from build123d import *

# Parameters (mm, degrees)
SKETCH1_W           = 1.905
SKETCH1_H           = 10.16
BOSS_EXTRUDE2_DEPTH = 3.175
SKETCH2_R           = 1.27
CUT_EXTRUDE1_DEPTH  = 52.07


with BuildPart() as part:
    # Sketch1 → Boss-Extrude2 (new body)
    with BuildSketch(Plane(origin=(0, 0, 0), x_dir=(1, 0, 0), z_dir=(0, 1, 0))):
        Polygon((-1.5875, 25.4), (-1.5875, -25.4), (1.5875, -25.4), (1.5875, 25.4), (1.5875, 38.1), (-1.5875, 38.1), align=None)
        with Locations((0, 31.75)):
            Rectangle(SKETCH1_W, SKETCH1_H, mode=Mode.SUBTRACT)
    extrude(amount=BOSS_EXTRUDE2_DEPTH)

    # Sketch2 → Cut-Extrude1 (cut)
    with BuildSketch(Plane.XY.offset(25.4)):
        with Locations((0, 1.5875)):
            Circle(SKETCH2_R)
    extrude(amount=-CUT_EXTRUDE1_DEPTH, mode=Mode.SUBTRACT)


solid = part.part
CAD build for the part. Positions are in the model's coordinates, mm. A direction names the side the tool comes from. Round coordinates to 2 decimals unless told otherwise and drop trailing zeros. Order: outer loops, then holes, each group sorted by start corner. A loop starts at its lowest first (then second) coordinate and runs counter-clockwise, first axis right, second up. Notation, with made-up numbers: (83, 17.5) - (104, 17.5) arc R15 cw to (104, 24.5) - close; hole circle Ø4 at (-18, 88). An arc over 180 degrees is marked (long way). Return JSON: item names as keys, results as strings.
(1) Cut at B-B (z = 18.5). Give the cut face in (x, y) (1 decimal).
Answer key:
{"outline": "(-1.6, 0) - (1.6, 0) - (1.6, 3.2) - (-1.6, 3.2) - close; hole circle Ø2.5 at (0, 1.6)"}
(2) Wall check: probe 1 along X at (y, z) = (0.75, -14); probe 2 along Y at (x, z) = (0, 6.5) (1 decimal); probe 3 along X at (y, z) = (1.65, -8.5). Give the ranges that are in metal, low to high. Write a range as from..to.
Answer key:
{"probe 1": "x = -1.59..-0.95, 0.95..1.59", "probe 2": "y = 0..0.3, 2.9..3.2", "probe 3": "x = -1.59..-1.27, 1.27..1.59"}
(3) Cut at A-A (x = 0). State how many separate pieces and enclosed holes the cut face has, then the cut area to 3 significant figures.
Answer key:
{"separate pieces": "3", "enclosed holes": "0", "area": "37.1 mm^2"}
(4) Pin check, flat tip, straight feed: pin 1 Ø1 at (x, y) = (0.5, 1.5) entering from +Z. Stop position of the tip, or through.
Answer key:
{"pin 1": "stops at z = -26.67"}
(5) Pull direction Z, two halves, no side cores. Call faces 1 (the face through (0, 3.175, -7)), 2 (the face through (0, 2, -38.1)), 3 (the face through (-0.952, 2, -32)), 4 (the face through (-0.022, 0.154, 25.4)): +Z half, -Z half, draft (parallel to the pull), parting line (faces both ways), or undercut.
Answer key:
{"face 1": "draft", "face 2": "-Z half", "face 3": "undercut", "face 4": "+Z half"}
(6) Tool access for faces 5 (the face through (-0.28, 0.35, -0.27)), 6 (the face through (0, 2, -36.83)), 7 (the face through (1.588, 2, -6)): list every direction of +Z, -Z, +X, -X, +Y, -Y with a clear straight run to the whole face (end or side of a thin tool).
Answer key:
{"face 5": "+Z", "face 6": "+Y, -Y", "face 7": "+Z, -Z, +X, +Y, -Y"}
